from build123d import *

# Parameters (mm, degrees)
F0_W     = 50
F0_H     = 50
F1_DEPTH = 2
F3_DEPTH = 25


with BuildPart() as f1:
    # F0 (on Top) → F1 (new body)
    with BuildSketch(Plane.XY):
        with Locations((0.755886, 0.681318)):
            Rectangle(F0_W, F0_H)
    extrude(amount=F1_DEPTH)


with BuildPart() as f3:
    # F2 (on Top) → F3 (new body)
    with BuildSketch(Plane.XY):
        Polygon((7.885135, 12.183912), (-7.614865, 12.183912), (-7.614865, 6.183912), (-12.114865, 6.183912), (-12.114865, -8.816088), (-7.614865, -8.816088), (-7.614865, -14.816088), (7.885135, -14.816088), (7.885135, -8.816088), (12.385135, -8.816088), (12.385135, 6.183912), (7.885135, 6.183912), align=None)
    extrude(amount=F3_DEPTH)


with BuildPart() as f1_1:
    add(f1.part)

    # F4: cut F3
    add(f3.part, mode=Mode.SUBTRACT)


solid = f1_1.part
Can you work these out from the model? Positions are in its coordinate system, mm. A direction names the side the tool comes from. Give positions to 0.01 mm unless a question says otherwise; leave off trailing zeros. Order: outer loops, then holes, each group sorted by start corner. A loop starts at its lowest first (then second) coordinate and runs counter-clockwise, first axis right, second up. Notation, with made-up numbers: M 60,-31 L 108,-31 A21 cw 108,-18 Z; hole C 16,-14.75 d10. An arc over 180 degrees is marked long. One line per question, with ' | ' between items.
Item 1: Please list where these lines run through material, in increasing order: L1, parallel to Y at x = 4.5, z = 1.35; L2, parallel to X at y = 4.5, z = 1.8.
Answer block:
L1: y = -24.32 to -14.82, 12.18 to 25.68 | L2: x = -24.24 to -12.11, 12.39 to 25.76
Item 2: Suppose I cut it at C-C, the plane z = 1.2. Write out the boundary of the cut face in (x, y).
Answer block:
outline: M -24.24,-24.32 L 25.76,-24.32 L 25.76,25.68 L -24.24,25.68 Z; hole M -12.11,-8.82 L -7.61,-8.82 L -7.61,-14.82 L 7.89,-14.82 L 7.89,-8.82 L 12.39,-8.82 L 12.39,6.18 L 7.89,6.18 L 7.89,12.18 L -7.61,12.18 L -7.61,6.18 L -12.11,6.18 Z
Item 3: Suppose I cut it at A-A, the plane y = -1.5. Write out the boundary of the cut face in (x, z), then the cut area to 3 significant figures.
Answer block:
outline: M -24.24,0 L -12.11,0 L -12.11,2 L -24.24,2 Z; M 12.39,0 L 25.76,0 L 25.76,2 L 12.39,2 Z | area: 51.0 mm2
Item 4: Suppose I cut it at B-B, the plane x = -3. Write out the boundary of the cut face in (y, z), then the cut area to 3 significant figures.
Answer block:
outline: M -24.32,0 L -14.82,0 L -14.82,2 L -24.32,2 Z; M 12.18,0 L 25.68,0 L 25.68,2 L 12.18,2 Z | area: 46.0 mm2
Item 5: I'm going to push a flat-ended pin straight in: pin 1 Ø4 at (x, y) = (-15, 3) entering from -Z. Where does the tip first touch, or does it pass through?
Answer block:
pin 1: stops at z = 0
Item 6: We'd pull the mould along Y, two halves only. Please class faces 1 (the face through (-7.615, -12, 1)), 2 (the face through (0, -24.319, 1)), 3 (the face through (-11, 7, 0)): released by +Y, released by -Y, zero draft, split by the parting line, or undercut.
Answer block:
face 1: undercut | face 2: released by -Y | face 3: zero draft
Item 7: For faces 4 (the face through (10, -8.816, 1)), 5 (the face through (-24.244, 0, 1)), which set-ups out of +Z, -Z, +X, -X, +Y, -Y let a thin tool reach every point of the face, with its end or its side?
Answer block:
face 4: +Z, -Z | face 5: +Z, -Z, -X, +Y, -Y
